Design review of the part built by this model. Coordinates are the model's own, in mm. A direction names the side the tool comes from. Round coordinates to 2 decimals unless told otherwise and drop trailing zeros. Loops run counter-clockwise (first coordinate to the right, second up) from the corner with the lowest first, then second, coordinate; pieces in that order, holes last. Notation, with made-up numbers: M 13,46 L 39,46 A28 cw 39,73 Z; hole C 68.25,42.25 d3. An arc over 180 degrees is marked long. One line per item, written item: value. Start each with the question number.
Item 1: We need section B-B (z = 3.5). Write out the cut boundary in (x, y), then the cut area to 3 significant figures.
Item 2: We need section A-A (z = 1.75). Write out the cut boundary in (x, y).
Item 3: Clearance check with flat-ended pins moving along their axes: pin 1 (4 mm diameter, centred on y = 3, z = 5, fed in from -X); pin 2 (1 mm diameter, centred on x = -2.5, y = 0, fed in from +Z); pin 3 (4 mm diameter, centred on y = -1.5, z = 5, fed in from +X). State where each tip first meets the part, or that it passes through.
Item 4: For line 1 along Z through (x, y) = (-2.75, 1.25); line 2 along Z through (x, y) = (2, 3.25); line 3 along Y through (x, z) = (-2.25, 3.5), list the stretches that pass through material, from the lowest coordinate up.
Item 5: For faces 1 (the flat face through (0, 0, 7)), 2 (the flat face through (-3, 1, 2)), list the 3-axis set-ups (+Z, -Z, +X, -X, +Y, -Y) from which the entire face can be reached by the end or side of a thin tool; tool diameter is ignored.
from build123d import *

# Parameters (mm, degrees)
F0_R     = 2.95
F1_DEPTH = 7
F1_TAPER = 0.5
F0_R_2   = 4
F2_DEPTH = 2
F3_R     = 1


with BuildPart() as f1:
    # F0 (on Top) → F1 (new body)
    with BuildSketch(Plane.XY):
        Circle(F0_R)
    extrude(amount=F1_DEPTH, taper=F1_TAPER)

    # F0 (on Top) → F2 (join)
    with BuildSketch(Plane.XY):
        Circle(F0_R_2)
        Circle(F0_R, mode=Mode.SUBTRACT)
        Circle(F0_R)
    extrude(amount=F2_DEPTH)

    # F3
    f3_edges = [f1.edges().sort_by_distance(p)[0] for p in [
        (-4, 0, 0),
        (-2.888912, 0, 7),
    ]]
    fillet(f3_edges, radius=F3_R)


solid = f1.part
A:
1. outline: C 0,0 d5.84
1. area: 26.8 mm2
2. outline: C 0,0 d8
3. pin 1: x = -2.73
3. pin 2: z = 6.99
3. pin 3: x = 2.92
4. line 1: 0 to 2
4. line 2: 0.42 to 2
4. line 3: -1.86 to 1.86
5. face 1: +Z, +X, -X, +Y, -Y
5. face 2: +Z
